```python
from build123d import *

# Parameters (mm, degrees)
TD_SKETCH_R                           = 0.79248
TL_FEATURE_DEPTH                      = 21.0312
TDF_180_DEG_REV_SKETCH_W              = 1.60495996
TDF_180_DEG_REV_SKETCH_H              = 1.60495996
TDF_180_DEG_REV_FEATURE_DEPTH         = 22.061040395
ISA_20_180_DEG_REV_FEATURE_DEPTH      = 22.061040395
ISA_20_180_DEG_REV_FEATURE_DEPTH_BACK = 22.061040395
F_10BA_180_DEG_REV_FEATURE_DEPTH      = 22.061040395
F_10BA_180_DEG_REV_FEATURE_DEPTH_BACK = 22.061040395


with BuildPart() as part:
    # TD_sketch → TL_feature (new body)
    with BuildSketch(Plane(origin=(0, 0, 0), x_dir=(1, 0, 0), z_dir=(0, 1, 0))):
        with Locations(Location((0, 0, 0), (0, 0, 270))):
            Circle(TD_SKETCH_R)
    extrude(amount=TL_FEATURE_DEPTH)

    # TDF_180_DEG_REV_sketch → TDF_180_DEG_REV_feature (cut, through all)
    with BuildSketch(Plane(origin=(0, 0, 0), x_dir=(1, 0, 0), z_dir=(0, 1, 0))):
        with Locations((1.17839998, 0)):
            Rectangle(TDF_180_DEG_REV_SKETCH_W, TDF_180_DEG_REV_SKETCH_H)
    extrude(amount=TDF_180_DEG_REV_FEATURE_DEPTH, mode=Mode.SUBTRACT)

    # ISA_20_180_DEG_REV_sketch → ISA_20_180_DEG_REV_feature (cut, two sides: drawn at the far end of the back side and taken through both)
    with BuildSketch(Plane(origin=(0, 0, 0), x_dir=(0, 0, -1), z_dir=(1, 0, 0)).offset(-ISA_20_180_DEG_REV_FEATURE_DEPTH_BACK)):
        Polygon((-12.996080373, 73.27228267), (-3.784567997, 21.0312), (-0.0762, 0), (0.0762, 0), (3.784567997, 21.0312), (12.996080373, 73.27228267), (12.996080373, -32.821688483), (-12.996080373, -32.821688483), align=None)
    extrude(amount=ISA_20_180_DEG_REV_FEATURE_DEPTH + ISA_20_180_DEG_REV_FEATURE_DEPTH_BACK, mode=Mode.SUBTRACT)

    # 10BA_180_DEG_REV_sketch → 10BA_180_DEG_REV_feature (cut, two sides: drawn at the far end of the back side and taken through both)
    with BuildSketch(Plane.XY.offset(-F_10BA_180_DEG_REV_FEATURE_DEPTH_BACK)):
        Polygon((-53.632984634, 0), (-0.79248, 0), (-0.71628, 0), (-0.427914365, 0.050846642), (3.271487997, 21.0312), (12.447145333, 73.068938636), (90.829329802, 2.18375769), (24.749199835, -70.885180946), align=None)
    extrude(amount=F_10BA_180_DEG_REV_FEATURE_DEPTH + F_10BA_180_DEG_REV_FEATURE_DEPTH_BACK, mode=Mode.SUBTRACT)


solid = part.part
```
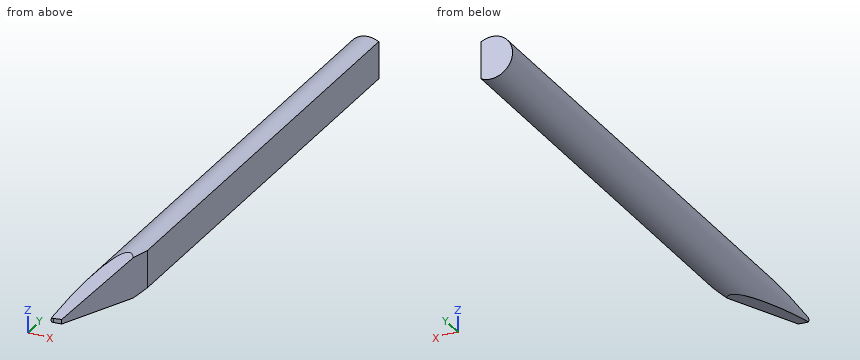
Geometry check sheet. Reference: the model listing, model coordinates, mm. Round coordinates to 2 decimals unless told otherwise and drop trailing zeros. Order: outer loops, then holes, each group sorted by start corner. A loop starts at its lowest first (then second) coordinate and runs counter-clockwise, first axis right, second up. Notation, with made-up numbers: (44.5, -39) - (49.5, -39) arc R18 ccw to (49.5, -19) - close; hole circle Ø7 at (-36.75, 59). An arc over 180 degrees is marked (long way). Use a Markdown table: item, result. Add a question column.
1) Section check D-D (y = 3.5). Record the cut outline in (x, z).
2) Section check B-B (y = 16.75). Record the cut outline in (x, z).
3) Section check C-C (z = 0.4). Record the cut outline in (x, y).
4) Thickness scan on line 1 along Z through (x, y) = (-0.65, 3.25); line 2 along Z through (x, y) = (-0.2, 7.75); line 3 along X through (y, z) = (18.25, 0.25). Record the ranges inside material, lowest first.
5) Section check A-A (x = 0). Record the cut outline in (y, z), then the cut area to 3 significant figures.
Established:
| question | item | result |
|---|---|---|
| 1 | outline | (-0.38, -0.69) - (0.18, -0.69) - (0.18, 0.69) - (-0.38, 0.69) arc R0.79 ccw to start |
| 2 | outline | (0.38, -0.7) - (0.38, 0.7) arc R0.79 ccw (long way) to start |
| 3 | outline | (-0.68, 1.84) - (-0.11, 1.84) - (0.38, 4.61) - (0.38, 21.03) - (-0.68, 21.03) - close |
| 4 | line 1 | -0.45 to 0.45 |
| 4 | line 2 | -0.77 to 0.77 |
| 4 | line 3 | -0.75 to 0.38 |
| 5 | outline | (2.48, -0.51) - (4.06, -0.79) - (21.03, -0.79) - (21.03, 0.79) - (4.06, 0.79) - (2.48, 0.51) - close |
| 5 | area | 29.0 mm2 |
